from build123d import *

# Parameters (mm, degrees)
SKETCH1_R           = 82.55
SKETCH1_R_2         = 2.54
SKETCH1_W           = 0.254
SKETCH1_H           = 25.4
SKETCH1_W_2         = 25.4
SKETCH1_H_2         = 0.254
BOSS_EXTRUDE1_DEPTH = 5.08


with BuildPart() as part:
    # Sketch1 → Boss-Extrude1 (new body)
    with BuildSketch(Plane(origin=(0, 0, 0), x_dir=(1, 0, 0), z_dir=(0, 1, 0))):
        with Locations(Location((0, 0, 0), (0, 0, 270))):
            Circle(SKETCH1_R)
        with Locations(Location((0, 0, 0), (0, 0, 270))):
            Circle(SKETCH1_R_2, mode=Mode.SUBTRACT)
        Polygon((13.327453739, 76.315109944), (13.577594908, 76.271003307), (9.166931196, 51.256886381), (8.916790026, 51.300993018), align=None, mode=Mode.SUBTRACT)
        with Locations((0, 64.77)):
            Rectangle(SKETCH1_W, SKETCH1_H, mode=Mode.SUBTRACT)
        Polygon((26.376959541, 72.84142389), (26.615641466, 72.754550774), (17.928329826, 48.886358206), (17.6896479, 48.973231323), align=None, mode=Mode.SUBTRACT)
        Polygon((38.625014774, 67.154488031), (38.844985226, 67.027488031), (26.144985226, 45.030442775), (25.925014774, 45.157442775), align=None, mode=Mode.SUBTRACT)
        Polygon((49.699468478, 59.427097035), (49.894043767, 59.263828982), (33.567238481, 39.806300127), (33.372663192, 39.96956818), align=None, mode=Mode.SUBTRACT)
        Polygon((59.263828982, 49.894043767), (59.427097035, 49.699468478), (39.96956818, 33.372663192), (39.806300127, 33.567238481), align=None, mode=Mode.SUBTRACT)
        Polygon((67.027488031, 38.844985226), (67.154488031, 38.625014774), (45.157442775, 25.925014774), (45.030442775, 26.144985226), align=None, mode=Mode.SUBTRACT)
        Polygon((72.754550774, 26.615641466), (72.84142389, 26.376959541), (48.973231323, 17.6896479), (48.886358206, 17.928329826), align=None, mode=Mode.SUBTRACT)
        Polygon((76.271003307, 13.577594908), (76.315109944, 13.327453739), (51.300993018, 8.916790026), (51.256886381, 9.166931196), align=None, mode=Mode.SUBTRACT)
        with Locations((64.77, 0)):
            Rectangle(SKETCH1_W_2, SKETCH1_H_2, mode=Mode.SUBTRACT)
        Polygon((76.315109944, -13.327453739), (76.271003307, -13.577594908), (51.256886381, -9.166931196), (51.300993018, -8.916790026), align=None, mode=Mode.SUBTRACT)
        Polygon((72.84142389, -26.376959541), (72.754550774, -26.615641466), (48.886358206, -17.928329826), (48.973231323, -17.6896479), align=None, mode=Mode.SUBTRACT)
        Polygon((67.154488031, -38.625014774), (67.027488031, -38.844985226), (45.030442775, -26.144985226), (45.157442775, -25.925014774), align=None, mode=Mode.SUBTRACT)
        Polygon((59.427097035, -49.699468478), (59.263828982, -49.894043767), (39.806300127, -33.567238481), (39.96956818, -33.372663192), align=None, mode=Mode.SUBTRACT)
        Polygon((49.894043767, -59.263828982), (49.699468478, -59.427097035), (33.372663192, -39.96956818), (33.567238481, -39.806300127), align=None, mode=Mode.SUBTRACT)
        Polygon((38.844985226, -67.027488031), (38.625014774, -67.154488031), (25.925014774, -45.157442775), (26.144985226, -45.030442775), align=None, mode=Mode.SUBTRACT)
        Polygon((26.615641466, -72.754550774), (26.376959541, -72.84142389), (17.6896479, -48.973231323), (17.928329826, -48.886358206), align=None, mode=Mode.SUBTRACT)
        Polygon((13.577594908, -76.271003307), (13.327453739, -76.315109944), (8.916790026, -51.300993018), (9.166931196, -51.256886381), align=None, mode=Mode.SUBTRACT)
        with Locations((0, -64.77)):
            Rectangle(SKETCH1_W, SKETCH1_H, mode=Mode.SUBTRACT)
        Polygon((-13.327453739, -76.315109944), (-13.577594908, -76.271003307), (-9.166931196, -51.256886381), (-8.916790026, -51.300993018), align=None, mode=Mode.SUBTRACT)
        Polygon((-26.376959541, -72.84142389), (-26.615641466, -72.754550774), (-17.928329826, -48.886358206), (-17.6896479, -48.973231323), align=None, mode=Mode.SUBTRACT)
        Polygon((-38.625014774, -67.154488031), (-38.844985226, -67.027488031), (-26.144985226, -45.030442775), (-25.925014774, -45.157442775), align=None, mode=Mode.SUBTRACT)
        Polygon((-49.699468478, -59.427097035), (-49.894043767, -59.263828982), (-33.567238481, -39.806300127), (-33.372663192, -39.96956818), align=None, mode=Mode.SUBTRACT)
        Polygon((-59.263828982, -49.894043767), (-59.427097035, -49.699468478), (-39.96956818, -33.372663192), (-39.806300127, -33.567238481), align=None, mode=Mode.SUBTRACT)
        Polygon((-67.027488031, -38.844985226), (-67.154488031, -38.625014774), (-45.157442775, -25.925014774), (-45.030442775, -26.144985226), align=None, mode=Mode.SUBTRACT)
        Polygon((-72.754550774, -26.615641466), (-72.84142389, -26.376959541), (-48.973231323, -17.6896479), (-48.886358206, -17.928329826), align=None, mode=Mode.SUBTRACT)
        Polygon((-76.271003307, -13.577594908), (-76.315109944, -13.327453739), (-51.300993018, -8.916790026), (-51.256886381, -9.166931196), align=None, mode=Mode.SUBTRACT)
        with Locations((-64.77, 0)):
            Rectangle(SKETCH1_W_2, SKETCH1_H_2, mode=Mode.SUBTRACT)
        Polygon((-76.315109944, 13.327453739), (-76.271003307, 13.577594908), (-51.256886381, 9.166931196), (-51.300993018, 8.916790026), align=None, mode=Mode.SUBTRACT)
        Polygon((-72.84142389, 26.376959541), (-72.754550774, 26.615641466), (-48.886358206, 17.928329826), (-48.973231323, 17.6896479), align=None, mode=Mode.SUBTRACT)
        Polygon((-67.154488031, 38.625014774), (-67.027488031, 38.844985226), (-45.030442775, 26.144985226), (-45.157442775, 25.925014774), align=None, mode=Mode.SUBTRACT)
        Polygon((-59.427097035, 49.699468478), (-59.263828982, 49.894043767), (-39.806300127, 33.567238481), (-39.96956818, 33.372663192), align=None, mode=Mode.SUBTRACT)
        Polygon((-49.894043767, 59.263828982), (-49.699468478, 59.427097035), (-33.372663192, 39.96956818), (-33.567238481, 39.806300127), align=None, mode=Mode.SUBTRACT)
        Polygon((-38.844985226, 67.027488031), (-38.625014774, 67.154488031), (-25.925014774, 45.157442775), (-26.144985226, 45.030442775), align=None, mode=Mode.SUBTRACT)
        Polygon((-26.615641466, 72.754550774), (-26.376959541, 72.84142389), (-17.6896479, 48.973231323), (-17.928329826, 48.886358206), align=None, mode=Mode.SUBTRACT)
        Polygon((-13.577594908, 76.271003307), (-13.327453739, 76.315109944), (-8.916790026, 51.300993018), (-9.166931196, 51.256886381), align=None, mode=Mode.SUBTRACT)
    extrude(amount=BOSS_EXTRUDE1_DEPTH)


solid = part.part
Input: part model. Units: mm. Frame: model coordinates. Give positions to 0.01 mm unless a question says otherwise; leave off trailing zeros. Write each loop counter-clockwise with the first axis right and the second up, starting at its lowest first coordinate (ties: lowest second). Pieces come first, ordered by that corner, then holes.
Q1. Section B-B, the plane x = 61.5. State how many separate pieces and enclosed holes the cut face has, plus the area to 3 significant figures.
Q2. Section C-C, the plane x = 42. Output: boundary loops of the cut face in (y, z).
Q3. First-contact query: P1, Ø2.5, axis at x = 62, y = 2.5, coming from the -Z side; P2, Ø1, axis at y = 1.5, z = 61, coming from the -X side; P3, Ø2.5, axis at y = 2, z = -68.5, coming from the -X side. Flat tips, straight axial feed; report the tip coordinate or a pass-through.
Q4. Section A-A, the plane z = 21. Output: boundary loops of the cut face in (x, y).
Q5. Material intervals for probe 1 along X at (y, z) = (3.2, 0); probe 2 along Z at (x, y) = (30, 2.45); probe 3 along X at (y, z) = (3.2, 28), sorted ascending.
Q6. Pull-direction query (Z, two-part tool) for faces 1 (the face through (22.21, 2.5, 60.65)), 2 (the face through (-17, 0, -1)), 3 (the face through (81.848, 2.504, -10.746)); classes: pulls with the +Z half, pulls with the -Z half, needs draft (parallel to the pull), parting line crosses it, or undercut.
Filled in:
1. separate pieces: 8
1. enclosed holes: 0
1. area: 550 mm2
2. outline: (0, -71.07) - (5.08, -71.07) - (5.08, -50.25) - (0, -50.25) - close; (0, -49.86) - (5.08, -49.86) - (5.08, -35.41) - (0, -35.41) - close; (0, -35.08) - (5.08, -35.08) - (5.08, 35.08) - (0, 35.08) - close; (0, 35.41) - (5.08, 35.41) - (5.08, 49.86) - (0, 49.86) - close; (0, 50.25) - (5.08, 50.25) - (5.08, 71.07) - (0, 71.07) - close
3. P1: stops at z = -55.89
3. P2: stops at x = -56.16
3. P3: stops at x = -47.87
4. outline: (-79.83, 0) - (-58.07, 0) - (-58.07, 5.08) - (-79.83, 5.08) - close; (-57.33, 0) - (57.33, 0) - (57.33, 5.08) - (-57.33, 5.08) - close; (58.07, 0) - (79.83, 0) - (79.83, 5.08) - (58.07, 5.08) - close
5. probe 1: x = -82.55 to -77.47, -52.07 to -2.54, 2.54 to 52.07, 77.47 to 82.55
5. probe 2: z = -76.91 to -52.22, -51.71 to 51.71, 52.22 to 76.91
5. probe 3: x = -77.66 to -48.75, -48.24 to 48.24, 48.75 to 77.66
6. face 1: undercut
6. face 2: needs draft
6. face 3: parting line crosses it
